```python
from build123d import *

# Parameters (mm, degrees)
SKETCH1_W           = 86
SKETCH1_H           = 55
BOSS_EXTRUDE1_DEPTH = 5
SKETCH2_R           = 7.5
CUT_EXTRUDE1_DEPTH  = 52.285962992
SKETCH3_W           = 66
SKETCH3_H           = 35
CUT_EXTRUDE2_DEPTH  = 52.285962992
FILLET1_R           = 2


with BuildPart() as part:
    # Sketch1 → Boss-Extrude1 (new body)
    with BuildSketch(Plane(origin=(0, 0, 0), x_dir=(1, 0, 0), z_dir=(0, 1, 0))):
        Rectangle(SKETCH1_W, SKETCH1_H)
    extrude(amount=BOSS_EXTRUDE1_DEPTH)

    # Sketch2 → Cut-Extrude1 (cut, through all)
    with BuildSketch(Plane(origin=(0, 5, 0), x_dir=(1, 0, 0), z_dir=(0, 1, 0))):
        with Locations(Location((19, -2.5, 0), (0, 0, 270))):
            Circle(SKETCH2_R)
    extrude(amount=-CUT_EXTRUDE1_DEPTH, mode=Mode.SUBTRACT)

    # Sketch3 → Cut-Extrude2 (cut, through all)
    with BuildSketch(Plane(origin=(0, 5, 0), x_dir=(1, 0, 0), z_dir=(0, 1, 0))):
        Rectangle(SKETCH3_W, SKETCH3_H)
    extrude(amount=-CUT_EXTRUDE2_DEPTH, mode=Mode.SUBTRACT)

    # Fillet1
    fillet1_edges = [part.edges().sort_by_distance(p)[0] for p in [
        (33, 2.5, -17.5),
        (33, 2.5, 17.5),
        (-33, 2.5, 17.5),
        (-33, 2.5, -17.5),
        (43, 2.5, 27.5),
        (-43, 2.5, 27.5),
        (-43, 2.5, -27.5),
        (43, 2.5, -27.5),
    ]]
    fillet(fillet1_edges, radius=FILLET1_R)


solid = part.part
```
Model file for the job. Use its own axes, mm. A direction names the side the tool comes from. Round coordinates to 2 decimals unless told otherwise and drop trailing zeros. Loops run counter-clockwise (first coordinate to the right, second up) from the corner with the lowest first, then second, coordinate; pieces in that order, holes last. Notation, with made-up numbers: M 2.25,-25.5 L 34.25,-25.5 A25 ccw 34.25,1.5 Z; hole C -22.5,-10.75 d11. An arc over 180 degrees is marked long. Put each result on its own line as item: value. Start each with the question number.
Item 1: Cut at C-C (y = 3.1). List the corners of the cut face in (x, z).
Item 2: Drill centre lines: line 1 along X through (y, z) = (0.9, -12); line 2 along Z through (x, y) = (29, 4.4); line 3 along X through (y, z) = (3.5, -16). Where is each one in solid material? Low to high.
Item 3: Cut at B-B (z = -16.5). List the corners of the cut face in (x, y).
Item 4: Mould opens along X. For faces 1 (the face through (33, 3, 0)), 2 (the face through (-1, 2, -27.5)), 3 (the face through (-43, 2, 0)) say: released by +X, released by -X, zero draft, split by the parting line, or undercut.
Item 5: Cut at A-A (x = 19). List the corners of the cut face in (y, z), then the cut area to 3 significant figures.
Item 6: 3-axis set-ups, long thin cutter, end or side, ignore diameter. For faces 4 (the face through (43, 2, 0)), 5 (the face through (-32.4, 2.46, 16.93)): which of +Z, -Z, +X, -X, +Y, -Y reach the whole face in a straight line?
Answer block:
1. outline: M -43,-25.5 A2 ccw -41,-27.5 L 41,-27.5 A2 ccw 43,-25.5 L 43,25.5 A2 ccw 41,27.5 L -41,27.5 A2 ccw -43,25.5 Z; hole M -33,-15.5 A2 ccw -31,-17.5 L 31,-17.5 A2 ccw 33,-15.5 L 33,15.5 A2 ccw 31,17.5 L -31,17.5 A2 ccw -33,15.5 Z
2. line 1: -43 to -33, 33 to 43
2. line 2: -27.5 to -17.5, 17.5 to 27.5
2. line 3: -43 to -32.94, 32.94 to 43
3. outline: M -43,0 L -32.73,0 L -32.73,5 L -43,5 Z; M 32.73,0 L 43,0 L 43,5 L 32.73,5 Z
4. face 1: undercut
4. face 2: zero draft
4. face 3: released by -X
5. outline: M 0,-27.5 L 5,-27.5 L 5,-17.5 L 0,-17.5 Z; M 0,17.5 L 5,17.5 L 5,27.5 L 0,27.5 Z
5. area: 100 mm2
6. face 4: +Z, -Z, +X, +Y, -Y
6. face 5: +Y, -Y
